Verification items for the finished model (mm, model axes). Face numbers are marked on the shaded views. A direction names the side the tool comes from. Round coordinates to 2 decimals unless told otherwise and drop trailing zeros. Order: outer loops, then holes, each group sorted by start corner. A loop starts at its lowest first (then second) coordinate and runs counter-clockwise, first axis right, second up.
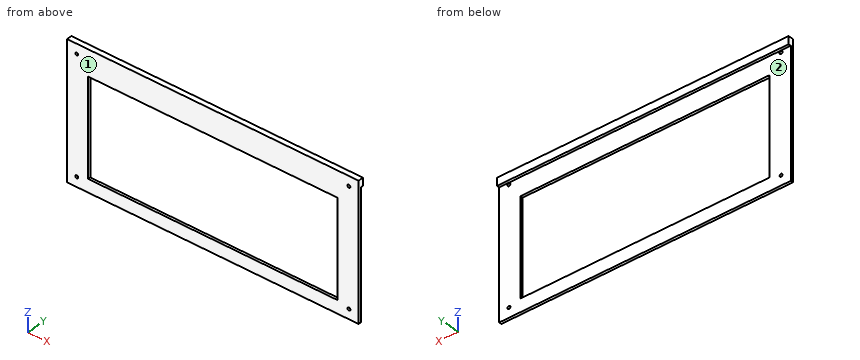
```python
from build123d import *

# Parameters (mm, degrees)
F_01_GUARD_OUTLINE_W      = 900
F_01_GUARD_OUTLINE_H      = 420
F_01_GUARD_OUTLINE_R      = 4.5
F_01_GUARD_OUTLINE_W_2    = 770
F_01_GUARD_OUTLINE_H_2    = 300
F_01_GUARD_PANEL_DEPTH    = 8
F_02_FRAME_RAIL_PROFILE_W = 900
F_02_FRAME_RAIL_PROFILE_H = 24
F_02_FRAME_RAIL_DEPTH     = 16


with BuildPart() as part:
    # 01_Guard_Outline → 01_Guard_Panel (new body)
    with BuildSketch(Plane(origin=(0, 0, 0), x_dir=(1, 0, 0), z_dir=(0, 1, 0))):
        Rectangle(F_01_GUARD_OUTLINE_W, F_01_GUARD_OUTLINE_H)
        with Locations(Location((-420, -180, 0), (0, 0, 270))):
            Circle(F_01_GUARD_OUTLINE_R, mode=Mode.SUBTRACT)
        with Locations(Location((420, -180, 0), (0, 0, 270))):
            Circle(F_01_GUARD_OUTLINE_R, mode=Mode.SUBTRACT)
        with Locations(Location((-420, 180, 0), (0, 0, 270))):
            Circle(F_01_GUARD_OUTLINE_R, mode=Mode.SUBTRACT)
        with Locations(Location((420, 180, 0), (0, 0, 270))):
            Circle(F_01_GUARD_OUTLINE_R, mode=Mode.SUBTRACT)
        with Locations((0, 20)):
            Rectangle(F_01_GUARD_OUTLINE_W_2, F_01_GUARD_OUTLINE_H_2, mode=Mode.SUBTRACT)
    extrude(amount=F_01_GUARD_PANEL_DEPTH)

    # 02_Frame_Rail_Profile → 02_Frame_Rail (add)
    with BuildSketch(Plane(origin=(0, 0, 0), x_dir=(1, 0, 0), z_dir=(0, 1, 0))):
        with Locations((0, -198)):
            Rectangle(F_02_FRAME_RAIL_PROFILE_W, F_02_FRAME_RAIL_PROFILE_H)
    extrude(amount=F_02_FRAME_RAIL_DEPTH)


solid = part.part
```
1) Sectioned sample at B-B on z = -61. Record the cut outline in (x, y).
2) Go/stop test with flat-tipped pins: pin 1 Ø10.5 at (x, z) = (420, 180) entering from +Y; pin 2 Ø9 at (x, y) = (-43.5, 13) entering from -Z; pin 3 Ø3 at (x, z) = (-175.5, 166) entering from -Y. Record where each tip stops, or that it passes through.
3) Sectioned sample at A-A on x = -151.5. Record the cut outline in (y, z), then the cut area to 3 significant figures.
4) Sectioned sample at C-C on z = 139. Record the cut outline in (x, y).
5) Tool access check on the marked faces 1 and 2. Record the directions out of +Z, -Z, +X, -X, +Y, -Y that give a thin tool (end or side, any length) a straight path to the whole face; none if there is none.
6) Scan lines: probe 1 along X at (y, z) = (6, -180); probe 2 along Z at (x, y) = (-420, 2.75); probe 3 along Z at (x, y) = (157, 3.25). Record each from-to range of solid material in increasing order.
Returned:
1. outline: (-450, 0) - (-385, 0) - (-385, 8) - (-450, 8) - close; (385, 0) - (450, 0) - (450, 8) - (385, 8) - close
2. pin 1: stops at y = 8
2. pin 2: stops at z = 186
2. pin 3: stops at y = 0
3. outline: (0, -210) - (8, -210) - (8, -170) - (0, -170) - close; (0, 130) - (8, 130) - (8, 186) - (16, 186) - (16, 210) - (0, 210) - close
3. area: 1,150 mm2
4. outline: (-450, 0) - (450, 0) - (450, 8) - (-450, 8) - close
5. face 1: +Z, -Z, +X, -X, -Y
5. face 2: -Z, +X, -X, +Y
6. probe 1: x = -450 to -424.5, -415.5 to 415.5, 424.5 to 450
6. probe 2: z = -210 to -184.5, -175.5 to 175.5, 184.5 to 210
6. probe 3: z = -210 to -170, 130 to 210
